Check sheet for the modelled part. Datum: model origin and axes. Units: mm. A direction names the side the tool comes from. Round coordinates to 2 decimals unless told otherwise and drop trailing zeros. Loops run counter-clockwise (first coordinate to the right, second up) from the corner with the lowest first, then second, coordinate; pieces in that order, holes last. Notation, with made-up numbers: (1, 46.5) - (58, 46.5) arc R10 cw to (58, 56.5) - close; hole circle Ø2 at (-17, 47.5). An arc over 180 degrees is marked (long way). Return JSON: item names as keys, results as strings.
from build123d import *

# Parameters (mm, degrees)
SALIENTE_EXTRUIR1_DEPTH = 16
SALIENTE_EXTRUIR2_DEPTH = 3
REDONDEO1_R             = 1.5


with BuildPart() as part:
    # Croquis1 → Saliente-Extruir1 (new body)
    with BuildSketch(Plane.XY):
        with BuildLine():
            Line((18.602755172, -8), (18.602755172, -10))
            Line((18.602755172, -10), (22.602755172, -10))
            Line((22.602755172, -10), (30, 22.25))
            Line((30, 22.25), (-30, 22.25))
            Line((-30, 22.25), (-22.602755172, -10))
            Line((-22.602755172, -10), (-18.602755172, -10))
            Line((-18.602755172, -10), (-18.602755172, -8))
            ThreePointArc((-18.602755172, -8), (0, 20.25), (18.602755172, -8))
        make_face()
    extrude(amount=SALIENTE_EXTRUIR1_DEPTH)

    # Croquis2 → Saliente-Extruir2 (add)
    with BuildSketch(Plane(origin=(0, 22.25, 0), x_dir=(1, 0, 0), z_dir=(0, 1, 0))):
        with BuildLine():
            Line((30, 0), (-30, 0))
            Line((-30, 0), (-36, 0))
            ThreePointArc((-36, 0), (-44, -8), (-36, -16))
            Line((-36, -16), (-30, -16))
            Line((-30, -16), (30, -16))
            Line((30, -16), (36, -16))
            ThreePointArc((36, -16), (44, -8), (36, 0))
            Line((36, 0), (30, 0))
        make_face()
        with BuildLine():
            Line((-37.5, -10.5), (-37.5, -5.5))
            ThreePointArc((-37.5, -5.5), (-36, -4), (-34.5, -5.5))
            Line((-34.5, -5.5), (-34.5, -10.5))
            ThreePointArc((-34.5, -10.5), (-36, -12), (-37.5, -10.5))
        make_face(mode=Mode.SUBTRACT)
        with BuildLine():
            Line((34.5, -10.5), (34.5, -5.5))
            ThreePointArc((34.5, -5.5), (36, -4), (37.5, -5.5))
            Line((37.5, -5.5), (37.5, -10.5))
            ThreePointArc((37.5, -10.5), (36, -12), (34.5, -10.5))
        make_face(mode=Mode.SUBTRACT)
    extrude(amount=SALIENTE_EXTRUIR2_DEPTH)

    # Redondeo1
    redondeo1_edges = [part.edges().sort_by_distance(p)[0] for p in [
        (-30, 22.25, 8),
        (30, 22.25, 8),
    ]]
    fillet(redondeo1_edges, radius=REDONDEO1_R)


solid = part.part
Q1. Sectioned sample at B-B (y = 5.5). Enter the section's corners in (x, z).
Answer key:
{"outline": "(-26.16, 0) - (-19.49, 0) - (-19.49, 16) - (-26.16, 16) - close; (19.49, 0) - (26.16, 0) - (26.16, 16) - (19.49, 16) - close"}
Q2. Depth check by flat-ended pin: P1, Ø1, axis at y = -9, z = 6.5, coming from the +X side; P2, Ø4, axis at x = -39, z = 11, coming from the -Y side; P3, Ø2.5, axis at y = 23.5, z = 9, coming from the -X side; P4, Ø4, axis at y = 15.5, z = 4, coming from the +X side. Enter the tip coordinate at first touch or a pass-through.
Answer key:
{"P1": "stops at x = 22.95", "P2": "stops at y = 22.25", "P3": "stops at x = -44", "P4": "stops at x = 28.91"}
Q3. Scan lines: probe 1 along X at (y, z) = (23.5, 9.5); probe 2 along Y at (x, z) = (0, 4.5); probe 3 along Y at (x, z) = (39, 3.5). Record each from-to range of solid material in increasing order. Write a range as [from, to].
Answer key:
{"probe 1": "x = [-43.86, -37.5], [-34.5, 34.5], [37.5, 43.86]", "probe 2": "y = [20.25, 25.25]", "probe 3": "y = [22.25, 25.25]"}
Q4. Sectioned sample at C-C (y = 0.5). Enter the section's corners in (x, z), plus the area to 3 significant figures.
Answer key:
{"outline": "(-25.01, 0) - (-20.24, 0) - (-20.24, 16) - (-25.01, 16) - close; (20.24, 0) - (25.01, 0) - (25.01, 16) - (20.24, 16) - close", "area": "153 mm²"}
Q5. Draft check along Z on faces 5 (the face through (3, 21, 0)), 6 (the face through (-36, 24, 12)), 7 (the face through (18.603, -9, 8)). Enter one of: released by +Z, released by -Z, zero draft, split by the parting line, or undercut.
Answer key:
{"face 5": "released by -Z", "face 6": "undercut", "face 7": "zero draft"}
Q6. Tool access check on faces 1 (the face through (37.5, 24, 8)), 2 (the face through (-18.603, -9, 8)), 3 (the face through (-38, 22.25, 8)), 4 (the face through (38, 22.25, 8)). Record the directions out of +Z, -Z, +X, -X, +Y, -Y that give a thin tool (end or side, any length) a straight path to the whole face; none if there is none.
Answer key:
{"face 1": "+Y, -Y", "face 2": "+Z, -Z, -Y", "face 3": "+Z, -Z, -X, -Y", "face 4": "+Z, -Z, +X, -Y"}
Q7. Sectioned sample at D-D (x = -11.5). Enter the section's corners in (y, z).
Answer key:
{"outline": "(16.67, 0) - (25.25, 0) - (25.25, 16) - (16.67, 16) - close"}
Q8. Sectioned sample at A-A (z = 8). Enter the section's corners in (x, y).
Answer key:
{"outline": "(-44, 22.25) - (-37.5, 22.25) - (-37.5, 25.25) - (-44, 25.25) - close; (-34.5, 22.25) - (-31.19, 22.25) arc R1.5 cw to (-29.73, 21.09) - (-22.6, -10) - (-18.6, -10) - (-18.6, -8) arc R20.25 cw (long way) to (18.6, -8) - (18.6, -10) - (22.6, -10) - (29.73, 21.09) arc R1.5 cw to (31.19, 22.25) - (34.5, 22.25) - (34.5, 25.25) - (-34.5, 25.25) - close; (37.5, 22.25) - (44, 22.25) - (44, 25.25) - (37.5, 25.25) - close"}
